Work out the finished part from the listing and answer in its coordinate system (mm). A direction names the side the tool comes from. Give positions to 0.01 mm unless a question says otherwise; leave off trailing zeros. Loops run counter-clockwise (first coordinate to the right, second up) from the corner with the lowest first, then second, coordinate; pieces in that order, holes last. Notation, with made-up numbers: M 34,16.5 L 45,16.5 A15 ccw 45,24.5 Z; hole C 25.5,27.25 d10. An arc over 180 degrees is marked long. Use a Markdown table: item, result.
```python
from build123d import *

# Parameters (mm, degrees)
F1_DEPTH = 25


with BuildPart() as f1:
    # F0 (on Right) → F1 (new body)
    with BuildSketch(Plane.YZ):
        with BuildLine():
            ThreePointArc((-31.450262, 5.139706), (-27.3825, 0.113026), (-21.617982, 3.042966))
            Line((-21.617982, 3.042966), (-4.565023, 41.208058))
            ThreePointArc((-4.565023, 41.208058), (0, 44.168311), (4.565023, 41.208058))
            Line((4.565023, 41.208058), (22.977643, 0))
            Line((22.977643, 0), (24.072928, 0))
            Line((24.072928, 0), (5.478027, 41.616008))
            ThreePointArc((5.478027, 41.616008), (0, 45.168311), (-5.478027, 41.616008))
            Line((-5.478027, 41.616008), (-22.530987, 3.450915))
            ThreePointArc((-22.530987, 3.450915), (-27.173938, 1.091035), (-30.450262, 5.139706))
            Line((-30.450262, 5.139706), (-31.450262, 5.139706))
        make_face()
    extrude(amount=F1_DEPTH)


solid = f1.part
```
(1) A cutting plane is placed at D-D (y = -27.5). Write down the section's boundary in (x, z), and give its area (3 significant figures).
Entries:
| item | result |
|---|---|
| outline | M 0,0.14 L 25,0.14 L 25,1.17 L 0,1.17 Z |
| area | 25.9 mm² |
(2) A cutting plane is placed at A-A (z = 20.5). Write down the section's boundary in (x, y), and give its area (3 significant figures).
Entries:
| item | result |
|---|---|
| outline | M 0,-14.91 L 25,-14.91 L 25,-13.82 L 0,-13.82 Z; M 0,13.82 L 25,13.82 L 25,14.91 L 0,14.91 Z |
| area | 54.8 mm² |
(3) Which of the six approach directions +Z, -Z, +X, -X, +Y, -Y give full straight-line access (tool end or side, diameter ignored) to faces 1 (the flat face through (12.32, -13.21, 21.86)), 2 (the cylindrical face through (12.325, -27.097, 1.075))?
Entries:
| item | result |
|---|---|
| face 1 | -Z, +X, -X |
| face 2 | +Z, +X, -X |
(4) A cutting plane is placed at B-B (x = 9.75). Write down the section's boundary in (y, z), and give its area (3 significant figures).
Entries:
| item | result |
|---|---|
| outline | M -31.45,5.14 A5.14 ccw -21.62,3.04 L -4.57,41.21 A5 cw 4.57,41.21 L 22.98,0 L 24.07,0 L 5.48,41.62 A6 ccw -5.48,41.62 L -22.53,3.45 A4.14 cw -30.45,5.14 Z |
| area | 112 mm² |
(5) Given P1, Ø8, axis at x = 19, z = 25, coming from the -Y side; P2, Ø5, axis at x = 8.5, y = -10, coming from the +Z side; P3, Ø2, axis at x = 7.5, z = 9.5, coming from the +Y side; P4, Ø10, axis at y = -19.5, z = 13.5, coming from the -X side, each flat-ended and moving along its own axis, determine where each tip first touches the part or whether it passes through.
Entries:
| item | result |
|---|---|
| P1 | stops at y = -14.69 |
| P2 | stops at z = 37.09 |
| P3 | stops at y = 20.27 |
| P4 | stops at x = 0 |
(6) The mould has two halves that part along Y. Classify faces 3 (the cylindrical face through (12.325, 0.097, 45.168)), 4 (the flat face through (0, -12, 26)), 5 (the flat face through (12.325, 13.642, 20.892)): released by +Y, released by -Y, zero draft, split by the parting line, or undercut.
Entries:
| item | result |
|---|---|
| face 3 | split by the parting line |
| face 4 | zero draft |
| face 5 | undercut |
(7) Consider probe 1 along Y at (x, z) = (15.5, 32.5); probe 2 along Y at (x, z) = (16.5, 16); probe 3 along Z at (x, y) = (22.25, -15). Determine where each line is inside the solid, lowest interval first. Write a range as [from, to].
Entries:
| item | result |
|---|---|
| probe 1 | y = [-9.55, -8.46], [8.46, 9.55] |
| probe 2 | y = [-16.92, -15.83], [15.83, 16.92] |
| probe 3 | z = [17.85, 20.31] |
(8) A cutting plane is placed at C-C (y = 12). Write down the section's boundary in (x, z), and give its area (3 significant figures).
Entries:
| item | result |
|---|---|
| outline | M 0,24.57 L 25,24.57 L 25,27.02 L 0,27.02 Z |
| area | 61.3 mm² |
